Here's how the part is built. I have some questions about the finished solid (model axes, mm). A direction names the side the tool comes from. Round coordinates to 2 decimals unless told otherwise and drop trailing zeros. Loops run counter-clockwise (first coordinate to the right, second up) from the corner with the lowest first, then second, coordinate; pieces in that order, holes last. Notation, with made-up numbers: M -28.75,58 L 15.25,58 A26 cw 15.25,80 Z; hole C 4,12.5 d2. An arc over 180 degrees is marked long. Answer as a JSON object with one key per item and string values.
from build123d import *

# Parameters (mm, degrees)
DODANIE_WYCI_GNI_CIE6_DEPTH = 18.5
SKORUPA2_T                  = -2
FILLET1_R                   = 5


with BuildPart() as part:
    # Szkic5 → Dodanie-wyciągnięcie6 (new body)
    with BuildSketch(Plane.XY):
        Polygon((38, 36.5), (51.5, 36.5), (51.5, -36.5), (-51.5, -36.5), (-51.5, 36.5), (-5.5, 36.5), align=None)
    extrude(amount=-DODANIE_WYCI_GNI_CIE6_DEPTH)

    # Skorupa2
    skorupa2_openings = [part.faces().sort_by_distance(p)[0] for p in [
        (0, 0, -18.5),
    ]]
    offset(amount=SKORUPA2_T, openings=skorupa2_openings, kind=Kind.INTERSECTION)

    # Fillet1
    fillet1_edges = [part.edges().sort_by_distance(p)[0] for p in [
        (51.5, -36.5, -9.25),
        (-51.5, -36.5, -9.25),
        (-51.5, 36.5, -9.25),
        (51.5, 36.5, -9.25),
    ]]
    fillet(fillet1_edges, radius=FILLET1_R)


solid = part.part
Item 1: I'm going to push a flat-ended pin straight in: pin 1 Ø3 at (x, y) = (-31.5, -16) entering from -Z. Where does the tip first touch, or does it pass through?
Resolved:
{"pin 1": "z = -2"}
Item 2: On a 3-axis mill with a long thin cutter (end or side, diameter ignored), from which of +Z, -Z, +X, -X, +Y, -Y can I reach the whole of each face in a straight line? I mean faces 1 (the face through (1, 1, 0)), 2 (the face through (1, 34.5, -10)). Say none if no direction works.
Resolved:
{"face 1": "+Z, +X, -X, +Y, -Y", "face 2": "-Z"}
Item 3: I want a section at B-B, the plane x = -4. Please give me the cut outline in (y, z).
Resolved:
{"outline": "M -36.5,-18.5 L -34.5,-18.5 L -34.5,-2 L 34.5,-2 L 34.5,-18.5 L 36.5,-18.5 L 36.5,0 L -36.5,0 Z"}
Item 4: I want a section at C-C, the plane y = -1.5. Please give me the cut outline in (x, z).
Resolved:
{"outline": "M -51.5,-18.5 L -49.5,-18.5 L -49.5,-2 L 49.5,-2 L 49.5,-18.5 L 51.5,-18.5 L 51.5,0 L -51.5,0 Z"}
Item 5: I want a section at A-A, the plane z = -15. Please give me the cut outline in (x, y), then the cut area to 3 significant figures.
Resolved:
{"outline": "M -51.5,-31.5 A5 ccw -46.5,-36.5 L 46.5,-36.5 A5 ccw 51.5,-31.5 L 51.5,31.5 A5 ccw 46.5,36.5 L -46.5,36.5 A5 ccw -51.5,31.5 Z; hole M -49.5,-34.5 L 49.5,-34.5 L 49.5,34.5 L -49.5,34.5 Z", "area": "667 mm²"}
Item 6: If we mould it in two halves opening along Y, with no side actions, what happens to faces 3 (the face through (-50, -35.07, -9.38)), 4 (the face through (1, -34.5, -10)), 5 (the face through (-51.5, 0, -9)), 6 (the face through (-49.5, 0, -10))? For each: pulls with the +Y half, pulls with the -Y half, needs draft (parallel to the pull), parting line crosses it, or undercut.
Resolved:
{"face 3": "pulls with the -Y half", "face 4": "undercut", "face 5": "needs draft", "face 6": "undercut"}
Item 7: Please list where these lines run through material, in increasing order: probe 1 along Y at (x, z) = (-32, -17); probe 2 along X at (y, z) = (7, -12.75); probe 3 along Z at (x, y) = (-31, 8). Write a range as from..to.
Resolved:
{"probe 1": "-36.5..-34.5, 34.5..36.5", "probe 2": "-51.5..-49.5, 49.5..51.5", "probe 3": "-2..0"}
